Input: part model. Units: mm. Frame: model coordinates. Face numbers are marked on the shaded views. A direction names the side the tool comes from. Give positions to 0.01 mm unless a question says otherwise; leave off trailing zeros. Loops run counter-clockwise (first coordinate to the right, second up) from the corner with the lowest first, then second, coordinate; pieces in that order, holes last. Notation, with made-up numbers: (42, -27.75) -> (66, -27.75) arc R27 cw to (66, 4.25) -> close; hole circle Ø9 at (-12, -5.5). An arc over 180 degrees is marked (long way). Answer as a JSON object with one key per item and string values.
```python
from build123d import *

# Parameters (mm, degrees)
BOSS_EXTRUDE1_DEPTH     = 8
CUT_EXTRUDE1_DEPTH      = 15.866068747
CUT_EXTRUDE1_DEPTH_BACK = 15.866068747
SKETCH3_W               = 7.7
SKETCH3_H               = 1.196323822
BOSS_EXTRUDE2_DEPTH     = 8
CHAMFER1_SIZE           = 1
FILLET1_R               = 1
SKETCH4_R               = 1.25
CUT_EXTRUDE2_DEPTH      = 16.387887332
CUT_EXTRUDE3_START      = 3
SKETCH5_R               = 2.25
CUT_EXTRUDE3_DEPTH      = 10
FILLET2_R               = 2
FILLET3_R               = 1
CHAMFER2_SIZE           = 1


# Some blends are built 0.0001 mm under size
with BuildPart() as part:
    # Sketch1 → Boss-Extrude1 (new body)
    with BuildSketch(Plane.XY):
        with BuildLine():
            Line((-3.3, 0), (-11, 0))
            Line((-11, 0), (-11, 6))
            Line((-11, 6), (11, 6))
            Line((11, 6), (11, 0))
            Line((11, 0), (3.3, 0))
            ThreePointArc((3.3, 0), (0, 3.3), (-3.3, 0))
        make_face()
    extrude(amount=BOSS_EXTRUDE1_DEPTH)

    # Sketch2 → Cut-Extrude1 (cut, two sides: drawn at the far end of the back side and taken through both)
    with BuildSketch(Plane.XY.offset(8).offset(-CUT_EXTRUDE1_DEPTH_BACK)):
        Polygon((-8.355690819, 4.422930452), (0, 6), (-11, 6), (-11, 1.504439372), align=None)
        Polygon((11, 6), (0, 6), (8.355690819, 4.422930452), (11, 1.504439372), align=None)
    extrude(amount=CUT_EXTRUDE1_DEPTH + CUT_EXTRUDE1_DEPTH_BACK, mode=Mode.SUBTRACT)

    # Sketch3 → Boss-Extrude2 (add)
    with BuildSketch(Plane.XY.offset(8)):
        with Locations((-7.15, -0.598161911)):
            Rectangle(SKETCH3_W, SKETCH3_H)
        with Locations((7.15, -0.598161911)):
            Rectangle(SKETCH3_W, SKETCH3_H)
    extrude(amount=-BOSS_EXTRUDE2_DEPTH)

    # Chamfer1
    chamfer1_edges = [part.edges().sort_by_distance(p)[0] for p in [
        (11, 0.154057775, 8),
        (-11, 0.154057775, 0),
        (-11, 0.154057775, 8),
        (11, 0.154057775, 0),
    ]]
    chamfer(chamfer1_edges, length=CHAMFER1_SIZE)

    # Fillet1
    fillet1_edges = [part.edges().sort_by_distance(p)[0] for p in [
        (-3.3, -1.196323822, 4),
        (3.3, -1.196323822, 4),
    ]]
    fillet(fillet1_edges, radius=FILLET1_R)

    # Sketch4 → Cut-Extrude2 (cut, through all)
    with BuildSketch(Plane.XZ.offset(1.196323822)):
        with Locations(Location((-5.25, 2.5, 0), (0, 0, 319.464197889))):
            Circle(SKETCH4_R)
        with Locations((5.25, 2.5)):
            Circle(SKETCH4_R)
    extrude(amount=-CUT_EXTRUDE2_DEPTH, mode=Mode.SUBTRACT)

    # Sketch5 → Cut-Extrude3 (cut)
    with BuildSketch(Plane(origin=(0, 0, 0), x_dir=(1, 0, 0), z_dir=(0, 1, 0)).offset(CUT_EXTRUDE3_START)):
        with Locations(Location((-5.25, -2.5, 0), (0, 0, 180))):
            Circle(SKETCH5_R)
        with Locations((5.25, -2.5)):
            Circle(SKETCH5_R)
    extrude(amount=CUT_EXTRUDE3_DEPTH, mode=Mode.SUBTRACT)

    # Fillet2
    fillet2_edges = [part.edges().sort_by_distance(p)[0] for p in [
        (8.355690819, 4.422930452, 4),
        (-8.355690819, 4.422930452, 4),
        (0, 6, 4),
        (-11, 1.504439372, 4),
    ]]
    fillet(fillet2_edges, radius=FILLET2_R)

    # Fillet3
    fillet3_edges = [part.edges().sort_by_distance(p)[0] for p in [
        (11, -1.196323822, 4),
        (-11, -1.196323822, 4),
    ]]
    fillet(fillet3_edges, radius=FILLET3_R)

    # Chamfer2
    chamfer2_edges = [part.edges().sort_by_distance(p)[0] for p in [
        (7.15, -1.196323822, 8),
        (3.592893219, -0.903430603, 8),
        (3.3, -0.098161911, 8),
        (0, 3.3, 8),
        (-3.3, -0.098161911, 8),
        (-3.592893219, -0.903430603, 8),
        (-7.15, -1.196323822, 8),
    ]]
    chamfer(chamfer2_edges, length=CHAMFER2_SIZE - 0.0001)  # a hair under: the kernel refuses the full size
    chamfer2_2_edges = [part.edges().sort_by_distance(p)[0] for p in [
        (7.15, -1.196323822, 0),
        (3.592893219, -0.903430603, 0),
        (3.3, -0.098161911, 0),
        (0, 3.3, 0),
        (-3.3, -0.098161911, 0),
        (-3.592893219, -0.903430603, 0),
        (-7.15, -1.196323822, 0),
    ]]
    chamfer(chamfer2_2_edges, length=CHAMFER2_SIZE - 0.0001)  # a hair under: the kernel refuses the full size
    # the kernel refuses this chamfer: 1 mm, written as the material it takes off along each edge
    with BuildSketch(Plane(origin=(8.806750236, 3.925101796, 0), x_dir=(-0.7407792072905057, -0.6711856247085939, -0.02749587661058639), z_dir=(0.6714394846228174, -0.7410593893133298, 0)), Plane(origin=(-11.7267295, 0.702357082, 0), x_dir=(0.7407792072905062, -0.6711856247085936, -0.02749587661058639), z_dir=(0.6714394846228171, 0.7410593893133303, 0))) as chamfer2_3_piece_1:
        with BuildLine():
            Line((1.028673195, 0), (-0.056547155, -1.027117794))
            Line((-0.056547155, -1.027117794), (-0.076539593, -1.026567876))
            ThreePointArc((-0.076539593, -1.026567876), (-0.034129227, -0.51339783), (-0.019992438, 0.000549918))
            Line((-0.019992438, 0.000549918), (0.000549918, 0.019992438))
            ThreePointArc((0.000549918, 0.019992438), (0.514497665, 0.00585565), (1.029223113, 0.019992438))
            Line((1.029223113, 0.019992438), (1.028673195, 0))
        make_face()
    extrude(amount=4.348834602, mode=Mode.SUBTRACT)
    with BuildSketch(Plane(origin=(7.324631458, 2.582222827, 0), x_dir=(0.7410593893133297, 0.6714394846228176, 0), z_dir=(0.6714394846228176, -0.7410593893133297, 0))) as chamfer2_3_piece_2:
        with BuildLine():
            Line((0.971715729, -0.028284271), (2.028284271, 1.028284271))
            Line((2.028284271, 1.028284271), (2.048284271, 1.028284271))
            ThreePointArc((2.048284271, 1.028284271), (2.02, 0.514142136), (2.02, 0))
            Line((2.02, 0), (2, -0.02))
            ThreePointArc((2, -0.02), (1.485857864, -0.02), (0.971715729, -0.048284271))
            Line((0.971715729, -0.048284271), (0.971715729, -0.028284271))
        make_face()
    revolve(axis=Axis((7.324631458, 2.582222827, 0), (0, 0, 1)), revolution_arc=37.133354948, mode=Mode.SUBTRACT)
    with BuildSketch(Plane(origin=(0.370934753, 5.929989044, 0), x_dir=(-0.18539725465470863, -0.9822788986514536, -0.02749587661058548), z_dir=(0.9826504221581788, -0.1854673767333577, 0)), Plane(origin=(-7.695566211, 4.547523671, 0), x_dir=(0.18539725465470863, -0.9822788986514536, -0.0274958766105855), z_dir=(0.9826504221581788, 0.1854673767333577, 0))) as chamfer2_3_piece_3:
        with BuildLine():
            Line((1.028673195, 0), (-0.056547155, -1.027117794))
            Line((-0.056547155, -1.027117794), (-0.076539593, -1.026567876))
            ThreePointArc((-0.076539593, -1.026567876), (-0.034129227, -0.51339783), (-0.019992438, 0.000549918))
            Line((-0.019992438, 0.000549918), (0.000549918, 0.019992438))
            ThreePointArc((0.000549918, 0.019992438), (0.514497665, 0.00585565), (1.029223113, 0.019992438))
            Line((1.029223113, 0.019992438), (1.028673195, 0))
        make_face()
    extrude(amount=7.45395442, mode=Mode.SUBTRACT)
    with BuildSketch(Plane(origin=(0, 3.964688199, 0), x_dir=(0.1854673767333581, 0.9826504221581787, 0), z_dir=(0.9826504221581787, -0.1854673767333581, 0))) as chamfer2_3_piece_4:
        with BuildLine():
            Line((0.971715729, -0.028284271), (2.028284271, 1.028284271))
            Line((2.028284271, 1.028284271), (2.048284271, 1.028284271))
            ThreePointArc((2.048284271, 1.028284271), (2.02, 0.514142136), (2.02, 0))
            Line((2.02, 0), (2, -0.02))
            ThreePointArc((2, -0.02), (1.485857864, -0.02), (0.971715729, -0.048284271))
            Line((0.971715729, -0.048284271), (0.971715729, -0.028284271))
        make_face()
    revolve(axis=Axis((0, 3.964688199, 0), (0, 0, 1)), revolution_arc=21.376765384, mode=Mode.SUBTRACT)
    with BuildSketch(Plane(origin=(-7.324631458, 2.582222827, 0), x_dir=(-0.1854673767333579, 0.9826504221581787, 0), z_dir=(0.9826504221581787, 0.1854673767333579, 0))) as chamfer2_3_piece_5:
        with BuildLine():
            Line((0.971715729, -0.028284271), (2.028284271, 1.028284271))
            Line((2.028284271, 1.028284271), (2.048284271, 1.028284271))
            ThreePointArc((2.048284271, 1.028284271), (2.02, 0.514142136), (2.02, 0))
            Line((2.02, 0), (2, -0.02))
            ThreePointArc((2, -0.02), (1.485857864, -0.02), (0.971715729, -0.048284271))
            Line((0.971715729, -0.048284271), (0.971715729, -0.028284271))
        make_face()
    revolve(axis=Axis((-7.324631458, 2.582222827, 0), (0, 0, 1)), revolution_arc=37.133354948, mode=Mode.SUBTRACT)
    # the kernel refuses this chamfer: 1 mm, written as the material it takes off along each edge
    with BuildSketch(Plane(origin=(8.806750236, 3.925101796, 8), x_dir=(-0.7407792072905057, -0.6711856247085939, 0.02749587661058564), z_dir=(0.6714394846228174, -0.7410593893133298, 0)), Plane(origin=(-11.7267295, 0.702357082, 8), x_dir=(0.740779207290506, -0.6711856247085934, 0.027495876610585612), z_dir=(0.6714394846228171, 0.7410593893133303, 0))) as chamfer2_4_piece_1:
        with BuildLine():
            Line((1.028673195, 0), (-0.056547155, 1.027117794))
            Line((-0.056547155, 1.027117794), (-0.076539593, 1.026567876))
            ThreePointArc((-0.076539593, 1.026567876), (-0.034129227, 0.51339783), (-0.019992438, -0.000549918))
            Line((-0.019992438, -0.000549918), (0.000549918, -0.019992438))
            ThreePointArc((0.000549918, -0.019992438), (0.514497665, -0.00585565), (1.029223113, -0.019992438))
            Line((1.029223113, -0.019992438), (1.028673195, 0))
        make_face()
    extrude(amount=4.348834602, mode=Mode.SUBTRACT)
    with BuildSketch(Plane(origin=(7.324631458, 2.582222827, 8), x_dir=(0.7410593893133297, 0.6714394846228176, 0), z_dir=(0.6714394846228176, -0.7410593893133297, 0))) as chamfer2_4_piece_2:
        with BuildLine():
            Line((0.971715729, 0.028284271), (2.028284271, -1.028284271))
            Line((2.028284271, -1.028284271), (2.048284271, -1.028284271))
            ThreePointArc((2.048284271, -1.028284271), (2.02, -0.514142136), (2.02, 0))
            Line((2.02, 0), (2, 0.02))
            ThreePointArc((2, 0.02), (1.485857864, 0.02), (0.971715729, 0.048284271))
            Line((0.971715729, 0.048284271), (0.971715729, 0.028284271))
        make_face()
    revolve(axis=Axis((7.324631458, 2.582222827, 8), (0, 0, 1)), revolution_arc=37.133354948, mode=Mode.SUBTRACT)
    with BuildSketch(Plane(origin=(0.370934753, 5.929989044, 8), x_dir=(-0.18539725465470863, -0.9822788986514536, 0.027495876610585605), z_dir=(0.9826504221581788, -0.1854673767333577, 0)), Plane(origin=(-7.695566211, 4.547523671, 8), x_dir=(0.18539725465470863, -0.9822788986514536, 0.02749587661058563), z_dir=(0.9826504221581788, 0.1854673767333577, 0))) as chamfer2_4_piece_3:
        with BuildLine():
            Line((1.028673195, 0), (-0.056547155, 1.027117794))
            Line((-0.056547155, 1.027117794), (-0.076539593, 1.026567876))
            ThreePointArc((-0.076539593, 1.026567876), (-0.034129227, 0.51339783), (-0.019992438, -0.000549918))
            Line((-0.019992438, -0.000549918), (0.000549918, -0.019992438))
            ThreePointArc((0.000549918, -0.019992438), (0.514497665, -0.00585565), (1.029223113, -0.019992438))
            Line((1.029223113, -0.019992438), (1.028673195, 0))
        make_face()
    extrude(amount=7.45395442, mode=Mode.SUBTRACT)
    with BuildSketch(Plane(origin=(0, 3.964688199, 8), x_dir=(0.1854673767333581, 0.9826504221581787, 0), z_dir=(0.9826504221581787, -0.1854673767333581, 0))) as chamfer2_4_piece_4:
        with BuildLine():
            Line((0.971715729, 0.028284271), (2.028284271, -1.028284271))
            Line((2.028284271, -1.028284271), (2.048284271, -1.028284271))
            ThreePointArc((2.048284271, -1.028284271), (2.02, -0.514142136), (2.02, 0))
            Line((2.02, 0), (2, 0.02))
            ThreePointArc((2, 0.02), (1.485857864, 0.02), (0.971715729, 0.048284271))
            Line((0.971715729, 0.048284271), (0.971715729, 0.028284271))
        make_face()
    revolve(axis=Axis((0, 3.964688199, 8), (0, 0, 1)), revolution_arc=21.376765384, mode=Mode.SUBTRACT)
    with BuildSketch(Plane(origin=(-7.324631458, 2.582222827, 8), x_dir=(-0.1854673767333579, 0.9826504221581787, 0), z_dir=(0.9826504221581787, 0.1854673767333579, 0))) as chamfer2_4_piece_5:
        with BuildLine():
            Line((0.971715729, 0.028284271), (2.028284271, -1.028284271))
            Line((2.028284271, -1.028284271), (2.048284271, -1.028284271))
            ThreePointArc((2.048284271, -1.028284271), (2.02, -0.514142136), (2.02, 0))
            Line((2.02, 0), (2, 0.02))
            ThreePointArc((2, 0.02), (1.485857864, 0.02), (0.971715729, 0.048284271))
            Line((0.971715729, 0.048284271), (0.971715729, 0.028284271))
        make_face()
    revolve(axis=Axis((-7.324631458, 2.582222827, 8), (0, 0, 1)), revolution_arc=37.133354948, mode=Mode.SUBTRACT)


solid = part.part
```
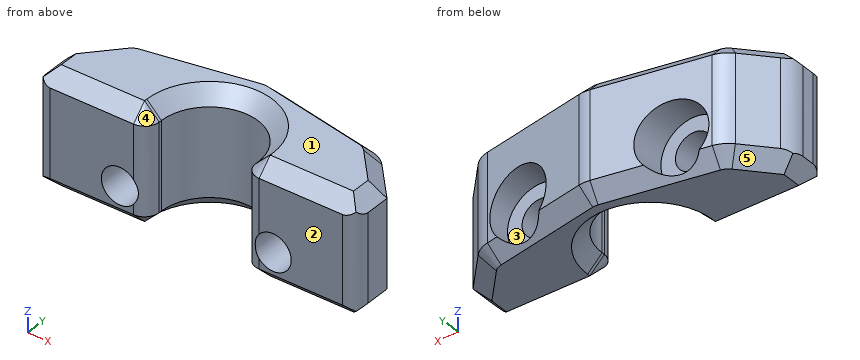
Q1. Pin query (flat end, axial travel): pin 1 (3.5 mm diameter, centred on x = -5.25, z = 2.5, fed in from +Y); pin 2 (2 mm diameter, centred on x = 6.5, z = 3.5, fed in from +Y). Return the tip coordinate at first contact, or that it passes through.
Evaluation:
{"pin 1": "stops at y = 3", "pin 2": "stops at y = 4.81"}
Q2. Section B-B, the plane z = 2.5. Give the number of separate pieces and of enclosed holes in the cut face, then the cut area to 3 significant figures.
Evaluation:
{"separate pieces": "3", "enclosed holes": "0", "area": "64.0 mm2"}
Q3. Ray query, line 1 along X through (y, z) = (3.5, 2.5); line 2 along Z through (x, y) = (-5.25, 1.3); line 3 along X through (y, z) = (3.6, 2.5). Return the intervals inside material, ascending.
Evaluation:
{"line 1": "x = -9.19 to -7.5, -3 to 3, 7.5 to 9.19", "line 2": "z = 0 to 1.25, 3.75 to 8", "line 3": "x = -9.1 to -7.5, -3 to 3, 7.5 to 9.1"}
Q4. Access query for the marked faces 4 and 5. Directions: +Z, -Z, +X, -X, +Y, -Y. A direction counts if a zero-diameter tool reaches every point of the face in a straight line with its end or side. Return the directions, or none.
Evaluation:
{"face 4": "+Z, -Y", "face 5": "-Z, -X, +Y"}
Q5. Draft query along Z for the marked faces 1, 2 and 3. Return one class per face: +Z half, -Z half, draft (parallel to the pull), parting line (faces both ways), or undercut.
Evaluation:
{"face 1": "+Z half", "face 2": "draft", "face 3": "undercut"}
Q6. Section C-C, the plane x = 5.25. Return the cut outline in (y, z), then the cut area to 3 significant figures.
Evaluation:
{"outline": "(-1.2, 1) -> (-0.2, 0) -> (3.99, 0) -> (4.25, 0.25) -> (3, 0.25) -> (3, 1.25) -> (-1.2, 1.25) -> close; (-1.2, 3.75) -> (3, 3.75) -> (3, 4.75) -> (5.01, 4.75) -> (5.01, 7) -> (3.99, 8) -> (-0.2, 8) -> (-1.2, 7) -> close", "area": "28.4 mm2"}
Q7. Section A-A, the plane z = 6. Return the cut outline in (x, y).
Evaluation:
{"outline": "(-11, -0.2) arc R1 ccw to (-10, -1.2) -> (-4.3, -1.2) arc R1 ccw to (-3.3, -0.2) -> (-3.3, 0) arc R3.3 cw to (3.3, 0) -> (3.3, -0.2) arc R1 ccw to (4.3, -1.2) -> (10, -1.2) arc R1 ccw to (11, -0.2) -> (11, 1.5) -> (8.81, 3.93) arc R2 ccw to (7.7, 4.55) -> (0.37, 5.93) arc R2 ccw to (-0.37, 5.93) -> (-7.7, 4.55) arc R2 ccw to (-8.81, 3.93) -> (-10.48, 2.08) arc R2 ccw to (-11, 0.73) -> close"}
